```python
from build123d import *

# Parameters (mm, degrees)
CROQUIS1_R              = 9
SALIENTE_EXTRUIR1_DEPTH = 12
REDONDEO1_R             = 30
CROQUIS2_R              = 5
CORTAR_EXTRUIR1_DEPTH   = 256.746915224
CROQUIS3_R              = 4.5
SALIENTE_EXTRUIR2_DEPTH = 12


with BuildPart() as part:
    # Croquis1 → Saliente-Extruir1 (new body)
    with BuildSketch(Plane.XY):
        with BuildLine():
            Line((24.517509814, 102.154502749), (221.020251881, 43.73046074))
            ThreePointArc((221.020251881, 43.73046074), (233.817531659, 20.103577105), (210.190648025, 7.306297327))
            Line((210.190648025, 7.306297327), (23.447731129, 62.828555729))
            Line((23.447731129, 62.828555729), (-209.97786522, 7.038852656))
            ThreePointArc((-209.97786522, 7.038852656), (-232.874076425, 21.101694207), (-218.811234874, 43.997905411))
            Line((-218.811234874, 43.997905411), (24.517509814, 102.154502749))
        make_face()
        with Locations((-214.394550047, 25.518379034)):
            Circle(CROQUIS1_R, mode=Mode.SUBTRACT)
        with Locations((215.605449953, 25.518379034)):
            Circle(CROQUIS1_R, mode=Mode.SUBTRACT)
    extrude(amount=SALIENTE_EXTRUIR1_DEPTH)

    # Redondeo1
    redondeo1_edges = [part.edges().sort_by_distance(p)[0] for p in [
        (23.447731129, 62.828555729, 6),
        (24.517509814, 102.154502749, 6),
    ]]
    fillet(redondeo1_edges, radius=REDONDEO1_R)

    # Croquis2 → Cortar-Extruir1 (cut, through all)
    with BuildSketch(Plane.XY.offset(12)):
        with Locations((138.923000663, 48.317545048)):
            Circle(CROQUIS2_R)
        with Locations((-97.681751872, 53.41323057)):
            Circle(CROQUIS2_R)
    extrude(amount=-CORTAR_EXTRUIR1_DEPTH, mode=Mode.SUBTRACT)

    # Croquis3 → Saliente-Extruir2 (add)
    with BuildSketch(Plane(origin=(0, 0, 0), x_dir=(-1, 0, 0), z_dir=(0, 0, -1))):
        with Locations(Location((-16.610214781, 89.982977062, 0), (0, 0, 180))):
            Circle(CROQUIS3_R)
    extrude(amount=SALIENTE_EXTRUIR2_DEPTH)


solid = part.part
```
Model file for the job. Use its own axes, mm. A direction names the side the tool comes from. Round coordinates to 2 decimals unless told otherwise and drop trailing zeros. Loops run counter-clockwise (first coordinate to the right, second up) from the corner with the lowest first, then second, coordinate; pieces in that order, holes last. Notation, with made-up numbers: M 53.5,22 L 74.5,22 A26 ccw 74.5,52 Z; hole C 11,-35.5 d10. An arc over 180 degrees is marked long. Put each result on its own line as item: value. Start each with the question number.
Item 1: Cut at A-A (z = 7.25). List the corners of the cut face in (x, y), then the cut area to 3 significant figures.
Item 2: Cut at C-C (y = 71.5). List the corners of the cut face in (x, z).
Item 3: Drill centre lines: line 1 along Z through (x, y) = (187.5, 30); line 2 along Y through (x, z) = (-64, 5.75); line 3 along Y through (x, z) = (-25, 5). Where is each one in solid material? Low to high.
Item 4: Mould opens along Y. For faces 4 (the face through (-232.772, 20.696, 5.916)), 5 (the face through (206.614, 25.914, 5.916)), 6 (the face through (24.599, 101.093, 6.084)), 7 (the face through (4, 65, 0)) say: released by +Y, released by -Y, zero draft, split by the parting line, or undercut.
Item 5: Drop flat-ended pins along their axis: P1, Ø2, axis at y = 37, z = 9, coming from the +X side; P2, Ø11.5, axis at x = -97.68, y = 53.41, coming from the -Z side. Give the stop position or say it passes through.
Item 6: Cut at B-B (x = 89.5). List the corners of the cut face in (y, z).
Item 7: 3-axis set-ups, long thin cutter, end or side, ignore diameter. For faces 1 (the face through (16.02, 85.52, -5.92)), 2 (the face through (-95.59, 34.38, 5.92)), 3 (the face through (-102.7, 71.75, 5.92)): which of +Z, -Z, +X, -X, +Y, -Y reach the whole face in a straight line?
Answer block:
1. outline: M -218.81,44 A19 ccw -209.98,7.04 L 15.63,60.96 A30 cw 31.15,60.54 L 210.19,7.31 A19 ccw 221.02,43.73 L 32.22,99.86 A30 ccw 16.7,100.29 Z; hole C -214.39,25.52 d18; hole C -97.68,53.41 d10; hole C 138.92,48.32 d10; hole C 215.61,25.52 d18
1. area: 17,400 mm2
2. outline: M -103.74,0 L 127.62,0 L 127.62,12 L -103.74,12 Z
3. line 1: 0 to 12
3. line 2: 41.93 to 81
3. line 3: 51.25 to 90.32
4. face 4: split by the parting line
4. face 5: undercut
4. face 6: released by +Y
4. face 7: zero draft
5. P1: x = 231.45
5. P2: z = 0
6. outline: M 43.19,0 L 82.83,0 L 82.83,12 L 43.19,12 Z
7. face 1: -Z
7. face 2: +Z, -Z, -Y
7. face 3: +Z, -Z, -X, +Y
